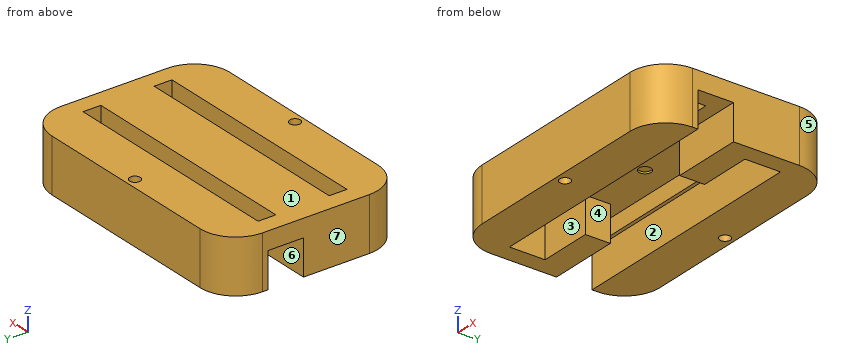
from build123d import *

# Parameters (mm, degrees)
SKETCH1_R           = 1.5
SKETCH1_W           = 65
SKETCH1_H           = 5
BOSS_EXTRUDE1_DEPTH = 15
CUT_EXTRUDE1_REACH  = 93.378
SKETCH2_W           = 10
SKETCH2_H           = 10
SKETCH3_W           = 35
SKETCH3_H           = 15
CUT_EXTRUDE2_DEPTH  = 10
SKETCH4_R           = 1.722798044
CUT_EXTRUDE3_DEPTH  = 0.5
SKETCH5_W           = 5
SKETCH5_H           = 10
BOSS_EXTRUDE2_DEPTH = 10


with BuildPart() as part:
    # Sketch1 → Boss-Extrude1 (new body)
    with BuildSketch(Plane.XY):
        with BuildLine():
            Line((10, 0), (65, 0))
            ThreePointArc((65, 0), (72.071067812, 2.928932188), (75, 10))
            Line((75, 10), (75, 40))
            ThreePointArc((75, 40), (72.071067812, 47.071067812), (65, 50))
            Line((65, 50), (10, 50))
            ThreePointArc((10, 50), (2.928932188, 47.071067812), (0, 40))
            Line((0, 40), (0, 10))
            ThreePointArc((0, 10), (2.928932188, 2.928932188), (10, 0))
        make_face()
        with Locations((37.5, 47.5)):
            Circle(SKETCH1_R, mode=Mode.SUBTRACT)
        with Locations((37.5, 2.5)):
            Circle(SKETCH1_R, mode=Mode.SUBTRACT)
        with Locations((37.5, 35)):
            Rectangle(SKETCH1_W, SKETCH1_H, mode=Mode.SUBTRACT)
        with Locations((37.5, 15)):
            Rectangle(SKETCH1_W, SKETCH1_H, mode=Mode.SUBTRACT)
    extrude(amount=BOSS_EXTRUDE1_DEPTH)

    # Cut-Extrude1: up to this face of the body (flat: up to its plane)
    cut_extrude1_end = Plane(part.part.faces().sort_by_distance((75, 25, 7.5))[0])
    # Sketch2 → Cut-Extrude1 (cut, up to the picked face)
    with BuildSketch(Plane.ZY, mode=Mode.PRIVATE) as cut_extrude1_sk1:
        with Locations((5, 33.5)):
            Rectangle(SKETCH2_W, SKETCH2_H)
    cut_extrude1_tool1 = split(extrude(cut_extrude1_sk1.sketch, amount=-CUT_EXTRUDE1_REACH, mode=Mode.PRIVATE), bisect_by=cut_extrude1_end, keep=Keep.BOTH, mode=Mode.PRIVATE)
    # Sketch2 → Cut-Extrude1 (cut, up to the picked face)
    with BuildSketch(Plane.ZY, mode=Mode.PRIVATE) as cut_extrude1_sk2:
        with Locations((5, 16.5)):
            Rectangle(SKETCH2_W, SKETCH2_H)
    cut_extrude1_tool2 = split(extrude(cut_extrude1_sk2.sketch, amount=-CUT_EXTRUDE1_REACH, mode=Mode.PRIVATE), bisect_by=cut_extrude1_end, keep=Keep.BOTH, mode=Mode.PRIVATE)
    add(cut_extrude1_tool1.solids().sort_by(Axis((0, 33.5, 5), (1, 0, 0)))[0], mode=Mode.SUBTRACT)
    add(cut_extrude1_tool2.solids().sort_by(Axis((0, 16.5, 5), (1, 0, 0)))[0], mode=Mode.SUBTRACT)

    # Sketch3 → Cut-Extrude2 (cut)
    with BuildSketch(Plane(origin=(0, 0, 0), x_dir=(-1, 0, 0), z_dir=(0, 0, -1))):
        with Locations((-37.5, 25)):
            Rectangle(SKETCH3_W, SKETCH3_H)
    extrude(amount=-CUT_EXTRUDE2_DEPTH, mode=Mode.SUBTRACT)

    # Sketch4 → Cut-Extrude3 (cut)
    with BuildSketch(Plane(origin=(0, 0, 10), x_dir=(-1, 0, 0), z_dir=(0, 0, -1))):
        with Locations(Location((-37.5, 25, 0), (0, 0, 90))):
            Circle(SKETCH4_R)
    extrude(amount=-CUT_EXTRUDE3_DEPTH, mode=Mode.SUBTRACT)

    # Sketch5 → Boss-Extrude2 (add)
    with BuildSketch(Plane(origin=(0, 0, 10), x_dir=(-1, 0, 0), z_dir=(0, 0, -1))):
        with Locations((-72.5, 33.5)):
            Rectangle(SKETCH5_W, SKETCH5_H)
        with Locations((-2.5, 16.5)):
            Rectangle(SKETCH5_W, SKETCH5_H)
    extrude(amount=BOSS_EXTRUDE2_DEPTH)


solid = part.part
The listing builds one solid part. Answer for the finished solid, in the listing's coordinates (mm). Face numbers are marked on the shaded views. A direction names the side the tool comes from. Round coordinates to 2 decimals unless told otherwise and drop trailing zeros. Loops run counter-clockwise (first coordinate to the right, second up) from the corner with the lowest first, then second, coordinate; pieces in that order, holes last. Notation, with made-up numbers: M 13,62 L 30,62 A17 cw 30,89 Z; hole C 60.25,89.5 d4. An arc over 180 degrees is marked long. Return JSON: item names as keys, results as strings.
Q1. Find section D-D, the plane x = 37.5. Determine the outline of the cut face in (y, z).
Results list:
{"outline": "M 0,0 L 1,0 L 1,15 L 0,15 Z; M 4,0 L 11.5,0 L 11.5,10 L 12.5,10 L 12.5,15 L 4,15 Z; M 17.5,10 L 23.28,10 L 23.28,10.5 L 26.72,10.5 L 26.72,10 L 32.5,10 L 32.5,15 L 17.5,15 Z; M 37.5,10 L 38.5,10 L 38.5,0 L 46,0 L 46,15 L 37.5,15 Z; M 49,0 L 50,0 L 50,15 L 49,15 Z"}
Q2. Which of the six approach directions +Z, -Z, +X, -X, +Y, -Y give full straight-line access (tool end or side, diameter ignored) to the marked faces 1, 2, 3 and 4?
Results list:
{"face 1": "+Z, +X, -X, +Y, -Y", "face 2": "-Z, -X", "face 3": "-Z, +X", "face 4": "-Z"}
Q3. Find the intervals of material crossed by line 1 along Y through (x, z) = (59, 11); line 2 along Y through (x, z) = (37.5, 11.5); line 3 along Y through (x, z) = (63.5, 5.25), in increasing order. Write a range as from..to.
Results list:
{"line 1": "y = 0..12.5, 17.5..32.5, 37.5..50", "line 2": "y = 0..1, 4..12.5, 17.5..32.5, 37.5..46, 49..50", "line 3": "y = 0..11.5, 21.5..28.5, 38.5..50"}
Q4. Find section A-A, the plane z = 1.5. Determine the outline of the cut face in (x, y), plus the area to 3 significant figures.
Results list:
{"outline": "M 0,10 A10 ccw 10,0 L 65,0 A10 ccw 75,10 L 75,11.5 L 5,11.5 L 5,21.5 L 20,21.5 L 20,28.5 L 0,28.5 Z; M 0,38.5 L 70,38.5 L 70,28.5 L 55,28.5 L 55,21.5 L 75,21.5 L 75,40 A10 ccw 65,50 L 10,50 A10 ccw 0,40 Z; hole C 37.5,2.5 d3; hole C 37.5,47.5 d3", "area": "2,010 mm2"}
Q5. Find section B-B, the plane y = 34.5. Determine the outline of the cut face in (x, z), plus the area to 3 significant figures.
Results list:
{"outline": "M 0,10 L 5,10 L 5,15 L 0,15 Z; M 70,0 L 75,0 L 75,15 L 70,15 Z", "area": "100 mm2"}
Q6. Find section C-C, the plane x = 64. Determine the outline of the cut face in (y, z).
Results list:
{"outline": "M 0,0 L 11.5,0 L 11.5,10 L 12.5,10 L 12.5,15 L 0,15 Z; M 17.5,10 L 21.5,10 L 21.5,0 L 28.5,0 L 28.5,10 L 32.5,10 L 32.5,15 L 17.5,15 Z; M 37.5,10 L 38.5,10 L 38.5,0 L 50,0 L 50,15 L 37.5,15 Z"}
Q7. Each of these flat-tipped pins is pushed along its axis until it touches: pin 1 Ø1 at (y, z) = (5.5, 6) entering from -X; pin 2 Ø8 at (x, y) = (47, 23.5) entering from -Z; pin 3 Ø1 at (x, z) = (66.5, 7) entering from +Y. Where does it stop, or does it pass through?
Results list:
{"pin 1": "stops at x = 0.83", "pin 2": "stops at z = 10", "pin 3": "stops at y = 49.95"}
Q8. The mould has two halves that part along Y. Classify the marked faces 5, 6 and 7: released by +Y, released by -Y, zero draft, split by the parting line, or undercut.
Results list:
{"face 5": "released by +Y", "face 6": "undercut", "face 7": "zero draft"}
